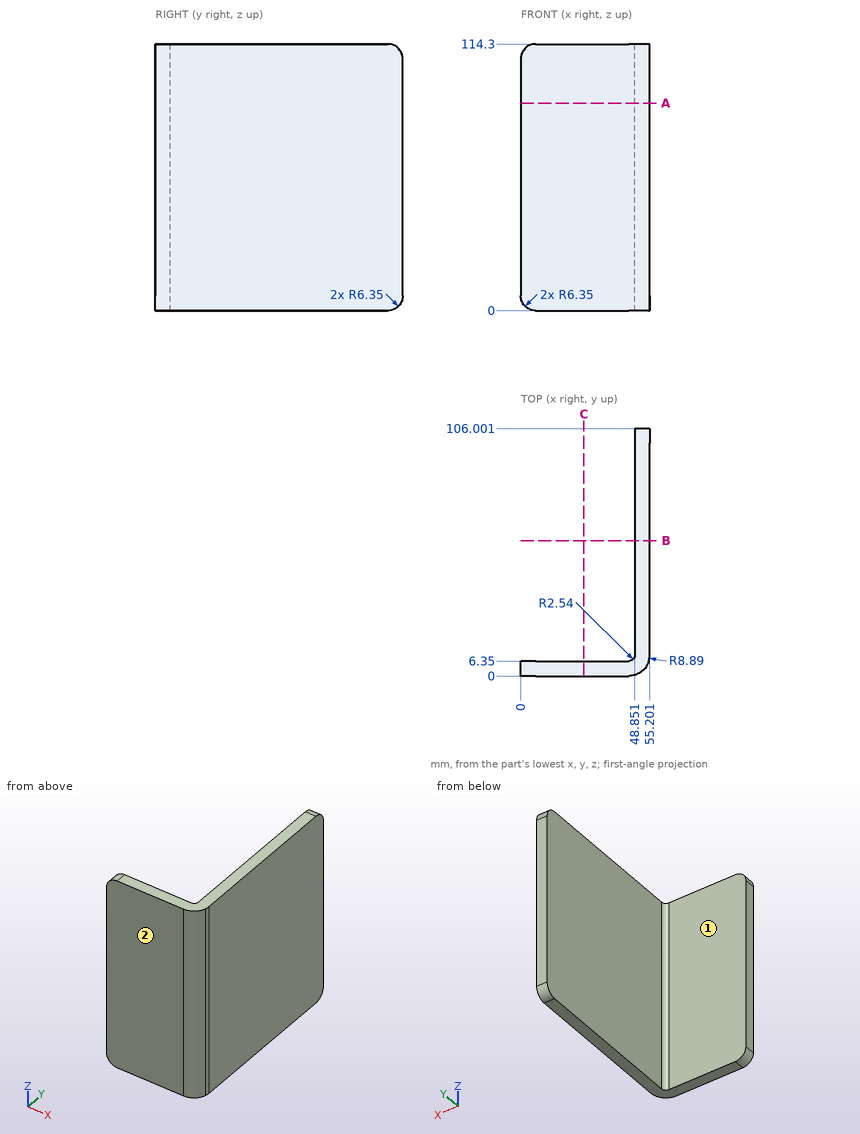
Geometry check sheet. Reference: drawing and pictorial views, mm from the part's lowest x, y, z. A direction names the side the tool comes from. Give positions to 0.01 mm unless a question says otherwise; leave off trailing zeros. Loops run counter-clockwise (first coordinate to the right, second up) from the corner with the lowest first, then second, coordinate; pieces in that order, holes last. Notation, with made-up numbers: M 47.25,-36 L 66.25,-36 A8 ccw 66.25,-22 Z; hole C 89,-17.75 d9. An arc over 180 degrees is marked long. Use a Markdown table: item, result. Add a question column.
Q1. Scan lines: line 1 along X through (y, z) = (28, 80); line 2 along Y through (x, z) = (13, 68.5); line 3 along Y through (x, z) = (51, 77) (1 decimal). Record each from-to range of solid material in increasing order. Write a range as [from, to].
Q2. Tool access check on the marked faces 1 and 2. Record the directions out of +Z, -Z, +X, -X, +Y, -Y that give a thin tool (end or side, any length) a straight path to the whole face; none if there is none.
Q3. Go/stop test with flat-tipped pins: pin 1 (23 mm diameter, centred on x = 26, z = 73.5, fed in from +Y); pin 2 (8 mm diameter, centred on y = 76, z = 29.5, fed in from -X). Record where each tip stops, or that it passes through.
Q4. Sectioned sample at B-B, the plane y = 58. Record the cut outline in (x, z).
Q5. Sectioned sample at C-C, the plane x = 27. Record the cut outline in (y, z), then the cut area to 3 significant figures.
Q6. Sectioned sample at A-A, the plane z = 89. Record the cut outline in (x, y).
Verdict:
| question | item | result |
|---|---|---|
| 1 | line 1 | [48.85, 55.2] |
| 1 | line 2 | [0, 6.35] |
| 1 | line 3 | [1.3, 106] |
| 2 | face 1 | +Z, -Z, -X, +Y |
| 2 | face 2 | +Z, -Z, +X, -X, -Y |
| 3 | pin 1 | y = 6.35 |
| 3 | pin 2 | x = 48.85 |
| 4 | outline | M 48.85,0 L 55.2,0 L 55.2,114.3 L 48.85,114.3 Z |
| 5 | outline | M 0,0 L 6.35,0 L 6.35,114.3 L 0,114.3 Z |
| 5 | area | 726 mm^2 |
| 6 | outline | M 0,0 L 46.31,0 A8.89 ccw 55.2,8.89 L 55.2,106 L 48.85,106 L 48.85,8.89 A2.54 cw 46.31,6.35 L 0,6.35 Z |
